Verification items for this drawing (mm, ordinates from the low corner). A direction names the side the tool comes from. Round coordinates to 2 decimals unless told otherwise and drop trailing zeros. Order: outer loops, then holes, each group sorted by start corner. A loop starts at its lowest first (then second) coordinate and runs counter-clockwise, first axis right, second up. Notation, with made-up numbers: M 71.5,-9 L 120.5,-9 A17 cw 120.5,24 Z; hole C -39.5,-36.75 d11. An arc over 180 degrees is marked long. Use CSV: the item, a comma, the result in double quotes. Start each with the question number.
Q1. Scan lines: line 1 (X direction, y = 33.5, z = 3.5); line 2 (Y direction, x = 7.5, z = 46.25); line 3 (Z direction, x = 24.25, y = 26). Record each from-to range of solid material in increasing order.
Q2. Gauge pin test, flat ends, axial feed: pin 1 Ø14 at (x, z) = (18.5, 4) entering from -Y; pin 2 Ø3 at (x, y) = (26, 5.5) entering from -Z; pin 3 Ø1.5 at (x, y) = (22.5, 33.5) entering from +Z; pin 4 Ø2.5 at (x, z) = (27, 23) entering from +Y. Record the tip position at first contact, or that the pin passes through.
Q3. Mould release check, pull along Y, two halves, no side actions. Record for the marked faces 4, 5 and 6: +Y half, -Y half, draft (parallel to the pull), parting line (faces both ways), or undercut.
Q4. Sectioned sample at C-C (y = 13). Enter the section's corners in (x, z).
Q5. Set-up check for the marked faces 1, 2 and 3: record each of +Z, -Z, +X, -X, +Y, -Y from which the full face is reachable in a straight line by a thin tool's end or side.
Q6. Sectioned sample at B-B (z = 26). Enter the section's corners in (x, y).
Q7. Sectioned sample at D-D (x = 11.75). Enter the section's corners in (y, z).
Q8. Sectioned sample at A-A (z = 44). Enter the section's corners in (x, y), and give its area (3 significant figures).
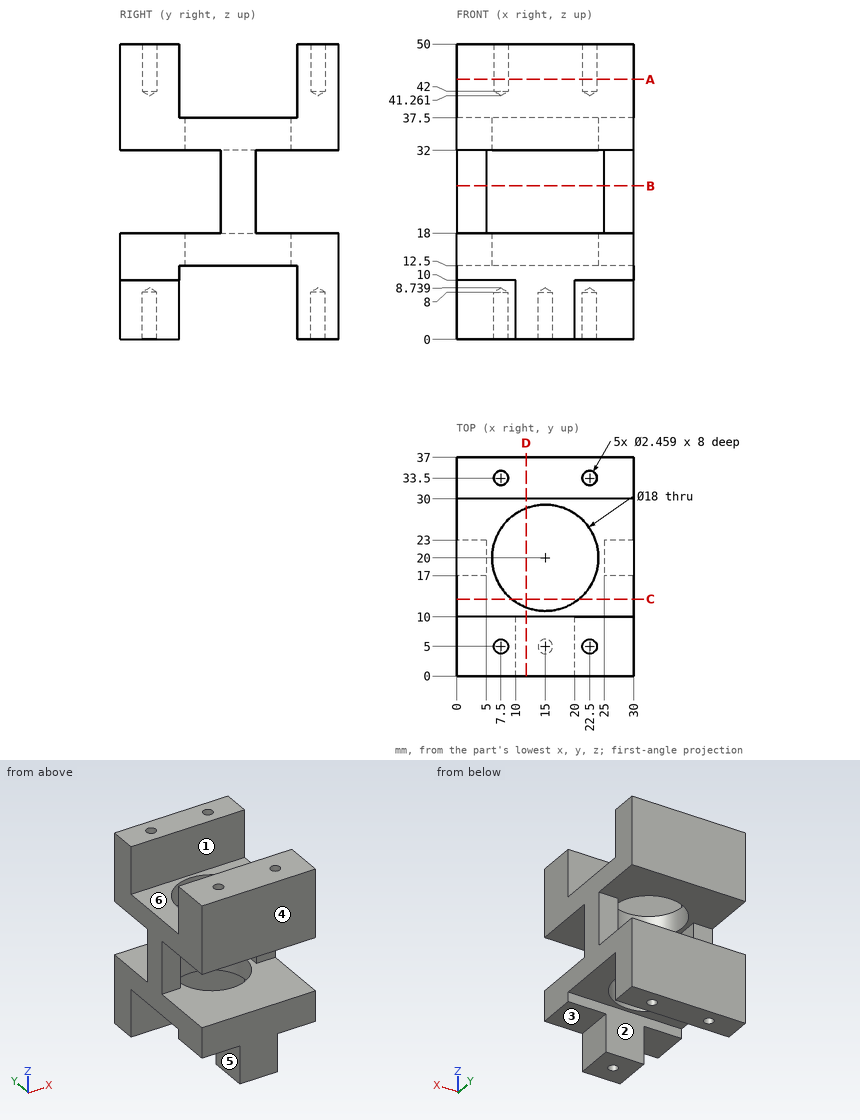
Verdict:
1,line 1,"x = 0 to 6.27, 8.73 to 21.27, 23.73 to 30"
1,line 2,"y = 0 to 3.77, 6.23 to 10, 30 to 32.27, 34.73 to 37"
1,line 3,"z = 12.5 to 18, 32 to 37.5"
2,pin 1,"stops at y = 0"
2,pin 2,"stops at z = 10"
2,pin 3,"stops at z = 41.71"
2,pin 4,"stops at y = 23"
3,face 4,"-Y half"
3,face 5,"draft"
3,face 6,"undercut"
4,outline,"M 0,12.5 L 9.34,12.5 L 9.34,18 L 0,18 Z; M 0,32 L 9.34,32 L 9.34,37.5 L 0,37.5 Z; M 20.66,12.5 L 30,12.5 L 30,18 L 20.66,18 Z; M 20.66,32 L 30,32 L 30,37.5 L 20.66,37.5 Z"
5,face 1,"+Z, +X, -X"
5,face 2,"-Z, +X, -X"
5,face 3,"-Z, +X, -Y"
6,outline,"M 0,17 L 5,17 L 5,23 L 0,23 Z; M 25,17 L 30,17 L 30,23 L 25,23 Z"
7,outline,"M 0,0 L 10,0 L 10,12.5 L 11.61,12.5 L 11.61,18 L 0,18 Z; M 0,32 L 11.61,32 L 11.61,37.5 L 10,37.5 L 10,50 L 0,50 Z; M 28.39,12.5 L 30,12.5 L 30,0 L 37,0 L 37,18 L 28.39,18 Z; M 28.39,32 L 37,32 L 37,50 L 30,50 L 30,37.5 L 28.39,37.5 Z"
8,outline,"M 0,0 L 30,0 L 30,10 L 0,10 Z; M 0,30 L 30,30 L 30,37 L 0,37 Z; hole C 7.5,5 d2.46; hole C 7.5,33.5 d2.46; hole C 22.5,5 d2.46; hole C 22.5,33.5 d2.46"
8,area,"491 mm²"
